Part model, mm, in its own coordinate system. A direction names the side the tool comes from. Coordinates: 2 decimals unless noted, no trailing zeros. Write each loop counter-clockwise with the first axis right and the second up, starting at its lowest first coordinate (ties: lowest second). Pieces come first, ordered by that corner, then holes. Notation, with made-up numbers: (61.25, 10.5) -> (99.25, 10.5) arc R24 ccw to (99.25, 23.5) -> close; hole circle Ø3 at (20, -10.5). An arc over 180 degrees is marked (long way). Write item = value, one per line. Start each with the question number.
Q1. Band-saw the part on A-A, the plane z = 8. List the corners of the cut face in (x, y), plus the area to 3 significant figures.
Q2. Tool access for faces 1 (the flat face through (14.8, 13.05, 7.9)), 2 (the flat face through (14.8, 22.05, 7.9)), 3 (the flat face through (6.427, 15, 7)), 4 (the flat face through (28.427, 15, 7)), 5 (the flat face through (14.8, 19.05, 7.9)): list every direction of +Z, -Z, +X, -X, +Y, -Y with a clear straight run to the whole face (end or side of a thin tool).
Q3. Pull direction Y, two halves, no side cores. Call faces 6 (the flat face through (17, 21, 14)), 7 (the flat face through (14.8, 16.05, 7.9)), 8 (the flat face through (17, 23.85, 1)): released by +Y, released by -Y, zero draft, split by the parting line, or undercut.
Q4. Band-saw the part on D-D, the plane x = 16.75. List the corners of the cut face in (y, z).
Q5. Band-saw the part on B-B, the plane y = 21.75. List the corners of the cut face in (x, z).
Q6. Pin check, flat tips, straight feed: P1, Ø0.9, axis at y = 20.5, z = 7, coming from the -X side; P2, Ø0.9, axis at y = 15.5, z = 9, coming from the +X side; P3, Ø5, axis at x = 14, z = 6, coming from the -Y side; P4, Ø4, axis at x = 17.43, z = 8, coming from the +Y side. Stop position of each tip, or through.
Q7. Probe line 1 (Y direction, x = 17.25, z = 13); line 2 (Z direction, x = 23, y = 16.75); line 3 (X direction, y = 13.75, z = 4). List the from-to ranges inside material, lowest first.
Q8. Band-saw the part on C-C, the plane z = 3. List the corners of the cut face in (x, y).
from build123d import *

# Parameters (mm, degrees)
F0_W     = 25.4
F0_H     = 12.7
F1_DEPTH = 2
F2_W     = 22
F2_H     = 3
F3_DEPTH = 12
F4_R     = 2.3
F5_DEPTH = 25
F6_R     = 2


with BuildPart() as f1:
    # F0 (on Top) → F1 (new body)
    with BuildSketch(Plane.XY):
        with Locations((17.427291, 17.500329)):
            Rectangle(F0_W, F0_H)
    extrude(amount=F1_DEPTH)

    # F2 (on face) → F3 (join)
    with BuildSketch(Plane.XY.offset(2)):
        with Locations((17.427291, 20.550329)):
            Rectangle(F2_W, F2_H)
        with Locations((17.427291, 14.550329)):
            Rectangle(F2_W, F2_H)
    extrude(amount=F3_DEPTH)

    # F4 (on face) → F5 (cut)
    with BuildSketch(Plane.XZ.offset(-13.050329)):
        with Locations((17.427291, 8)):
            Circle(F4_R)
    extrude(amount=-F5_DEPTH, mode=Mode.SUBTRACT)

    # F6
    f6_edges = [f1.edges().sort_by_distance(p)[0] for p in [
        (6.427291, 20.550329, 14),
        (6.427291, 14.550329, 14),
        (28.427291, 20.550329, 14),
        (28.427291, 14.550329, 14),
    ]]
    fillet(f6_edges, radius=F6_R)


solid = f1.part
Ans:
q1.outline = (6.43, 13.05) -> (15.13, 13.05) -> (15.13, 16.05) -> (6.43, 16.05) -> close; (6.43, 19.05) -> (15.13, 19.05) -> (15.13, 22.05) -> (6.43, 22.05) -> close; (19.73, 13.05) -> (28.43, 13.05) -> (28.43, 16.05) -> (19.73, 16.05) -> close; (19.73, 19.05) -> (28.43, 19.05) -> (28.43, 22.05) -> (19.73, 22.05) -> close
q1.area = 104 mm2
q2.face_1 = +Z, +X, -X, -Y
q2.face_2 = +Z, +X, -X, +Y
q2.face_3 = +Z, -X, +Y, -Y
q2.face_4 = +Z, +X, +Y, -Y
q2.face_5 = +Z, +X, -X
q3.face_6 = zero draft
q3.face_7 = undercut
q3.face_8 = released by +Y
q4.outline = (11.15, 0) -> (23.85, 0) -> (23.85, 2) -> (22.05, 2) -> (22.05, 5.8) -> (19.05, 5.8) -> (19.05, 2) -> (16.05, 2) -> (16.05, 5.8) -> (13.05, 5.8) -> (13.05, 2) -> (11.15, 2) -> close; (13.05, 10.2) -> (16.05, 10.2) -> (16.05, 14) -> (13.05, 14) -> close; (19.05, 10.2) -> (22.05, 10.2) -> (22.05, 14) -> (19.05, 14) -> close
q5.outline = (4.73, 0) -> (30.13, 0) -> (30.13, 2) -> (28.43, 2) -> (28.43, 12) arc R2 ccw to (26.43, 14) -> (8.43, 14) arc R2 ccw to (6.43, 12) -> (6.43, 2) -> (4.73, 2) -> close; hole circle Ø4.6 at (17.43, 8)
q6.P1 = 6.43
q6.P2 = 28.43
q6.P3 = 13.05
q6.P4 = through
q7.line_1 = 13.05 to 16.05, 19.05 to 22.05
q7.line_2 = 0 to 2
q7.line_3 = 6.43 to 28.43
q8.outline = (6.43, 13.05) -> (28.43, 13.05) -> (28.43, 16.05) -> (6.43, 16.05) -> close; (6.43, 19.05) -> (28.43, 19.05) -> (28.43, 22.05) -> (6.43, 22.05) -> close
